Job drawing, mm, ordinate dimensions from the low corner. One solid piece. A direction names the side the tool comes from. Give positions to 0.01 mm unless a question says otherwise; leave off trailing zeros. Loops run counter-clockwise (first coordinate to the right, second up) from the corner with the lowest first, then second, coordinate; pieces in that order, holes last. Notation, with made-up numbers: M -2,-39.5 L 23,-39.5 A21 cw 23,-33.5 Z; hole C 34.25,27.25 d6. An arc over 180 degrees is marked long. Answer as CSV lines item,"result".
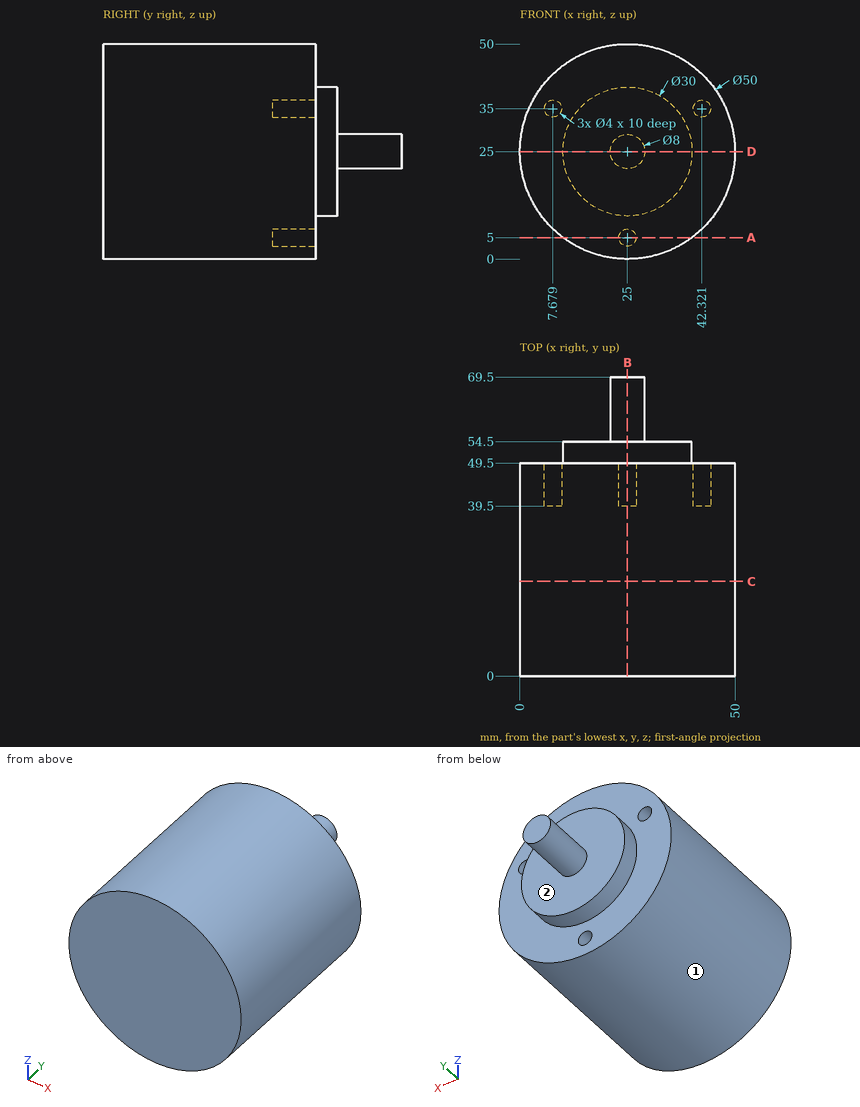
1) Band-saw the part on C-C on y = 22. Give the cut face in (x, z).
Answer below:
outline,"C 25,25 d50"
2) Which spindle directions (+Z, -Z, +X, -X, +Y, -Y) get a long thin tool onto all of the face, cutting with end or side? Do the marked faces 1 and 2. Say none if no direction does.
Answer below:
face 1,"+Y, -Y"
face 2,"+Y"
3) Drill centre lines: line 1 (X direction, y = 43, z = 35); line 2 (X direction, y = 43.5, z = 5); line 3 (Z direction, x = 25, y = 45.5). Where is each one in solid material? Low to high. Write a range as from..to.
Answer below:
line 1,"x = 2.09..5.68, 9.68..40.32, 44.32..47.91"
line 2,"x = 10..23, 27..40"
line 3,"z = 0..3, 7..50"
4) Band-saw the part on D-D on z = 25. Give the cut face in (x, y), and give its area (4 significant figures).
Answer below:
outline,"M 0,0 L 50,0 L 50,49.5 L 40,49.5 L 40,54.5 L 29,54.5 L 29,69.5 L 21,69.5 L 21,54.5 L 10,54.5 L 10,49.5 L 0,49.5 Z"
area,"2,745 mm^2"
5) Flat gauge pins, fed straight in: pin 1 (12 mm diameter, centred on y = 7.5, z = 43, fed in from -X); pin 2 (4 mm diameter, centred on x = 41.5, z = 20, fed in from -Y); pin 3 (1 mm diameter, centred on y = 18, z = 18, fed in from +X); pin 4 (3 mm diameter, centred on x = 42.5, z = 34, fed in from +Y). Where does each tip first touch, or does it go through?
Answer below:
pin 1,"stops at x = 3.07"
pin 2,"stops at y = 0"
pin 3,"stops at x = 49.14"
pin 4,"stops at y = 49.5"
6) Band-saw the part on B-B on x = 25. Give the cut face in (y, z).
Answer below:
outline,"M 0,0 L 49.5,0 L 49.5,3 L 39.5,3 L 39.5,7 L 49.5,7 L 49.5,10 L 54.5,10 L 54.5,21 L 69.5,21 L 69.5,29 L 54.5,29 L 54.5,40 L 49.5,40 L 49.5,50 L 0,50 Z"
7) Band-saw the part on A-A on z = 5. Give the cut face in (x, y).
Answer below:
outline,"M 10,0 L 40,0 L 40,49.5 L 27,49.5 L 27,39.5 L 23,39.5 L 23,49.5 L 10,49.5 Z"
